from build123d import *

# Parameters (mm, degrees)
BOSS_EXTRUDE1_DEPTH = 3.175
FILLET1_R           = 12.7
FILLET2_R           = 1.5875


with BuildPart() as part:
    # Sketch1 → Boss-Extrude1 (new body)
    with BuildSketch(Plane.XY):
        Polygon((2.921, 6.35), (2.921, 11.049), (9.271, 11.049), (9.271, 14.224), (41.021, 14.224), (41.021, 11.049), (11.901256121, 5.243743879), (6.096, -12.7), (2.921, -12.7), (2.921, -6.35), (-2.921, -6.35), (-2.921, 6.35), align=None)
    extrude(amount=BOSS_EXTRUDE1_DEPTH)

    # Fillet1
    fillet1_edges = [part.edges().sort_by_distance(p)[0] for p in [
        (11.901256121, 5.243743879, 1.5875),
    ]]
    fillet(fillet1_edges, radius=FILLET1_R)

    # Fillet2
    fillet2_edges = [part.edges().sort_by_distance(p)[0] for p in [
        (41.021, 11.049, 1.5875),
        (6.096, -12.7, 1.5875),
    ]]
    fillet(fillet2_edges, radius=FILLET2_R)


solid = part.part
Verification items for the finished model (mm, model axes). A direction names the side the tool comes from. Give positions to 0.01 mm unless a question says otherwise; leave off trailing zeros. Write each loop counter-clockwise with the first axis right and the second up, starting at its lowest first coordinate (ties: lowest second). Pieces come first, ordered by that corner, then holes. Notation, with made-up numbers: M -17.75,12 L -6.75,12 A14 cw -6.75,17 Z; hole C -29,4 d4. An arc over 180 degrees is marked long. Use CSV: the item, a comma, the result in double quotes.
1) Cross-section at B-B (x = 25). Enter the section's corners in (y, z) (3 decimals).
Final values:
outline,"M 7.855,0 L 14.224,0 L 14.224,3.175 L 7.855,3.175 Z"
2) Go/stop test with flat-tipped pins: pin 1 Ø2 at (x, y) = (19, 5.5) entering from +Z; pin 2 Ø1.5 at (x, z) = (2.5, 1.5) entering from +Y; pin 3 Ø1.6 at (x, z) = (1, 1.5) entering from -Y; pin 4 Ø1.5 at (y, z) = (1, 2.5) entering from +X. Record where each tip stops, or that it passes through.
Final values:
pin 1,"through"
pin 2,"y = 11.05"
pin 3,"y = -6.35"
pin 4,"x = 11.45"
3) Cross-section at C-C (y = -9). Enter the section's corners in (x, z) (3 decimals).
Final values:
outline,"M 2.921,0 L 7.293,0 L 7.293,3.175 L 2.921,3.175 Z"
4) Access from +Z, -Z, +X, -X, +Y, -Y to the whole of each face (thin tool, end or side, straight path). Record for faces 1 (the face through (29.62, 8.776, 1.565)), 2 (the face through (0, -6.35, 2)), 3 (the face through (2.921, 9, 2)).
Final values:
face 1,"+Z, -Z, +X, -Y"
face 2,"+Z, -Z, -X, -Y"
face 3,"+Z, -Z, -X, +Y"
5) Material ranges on line 1 along X through (y, z) = (12.5, 2.95); line 2 along Y through (x, z) = (5, 1.5); line 3 along Y through (x, z) = (0, 1.9), recorded low to high.
Final values:
line 1,"9.27 to 41.02"
line 2,"-12.7 to 11.05"
line 3,"-6.35 to 6.35"
